```python
from build123d import *

# Parameters (mm, degrees)
F0_W     = 100
F0_H     = 100
F1_DEPTH = 100
F2_W     = 100
F2_H     = 20
F3_DEPTH = 40
F4_W     = 60.561549
F4_H     = 32.747179
F5_DEPTH = 100.001


with BuildPart() as f1:
    # F0 (on Top) → F1 (new body)
    with BuildSketch(Plane.XY):
        Rectangle(F0_W, F0_H)
    extrude(amount=F1_DEPTH)

    # F2 (on face) → F3 (join)
    with BuildSketch(Plane.XY.offset(100)):
        with Locations((0, 40)):
            Rectangle(F2_W, F2_H)
    extrude(amount=F3_DEPTH)

    # F4 (on face) → F5 (cut, through all)
    with BuildSketch(Plane.XZ.offset(50)):
        with Locations((-2.157872, 16.373589)):
            Rectangle(F4_W, F4_H)
    extrude(amount=-F5_DEPTH, mode=Mode.SUBTRACT)


solid = f1.part
```
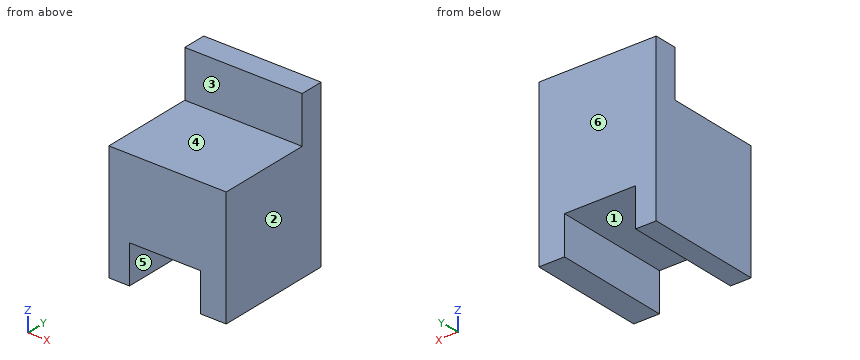
The model under review builds one solid part; all positions refer to its coordinate system, in mm. Face numbers are marked on the shaded views. A direction names the side the tool comes from. Coordinates: 2 decimals unless noted, no trailing zeros. Write each loop counter-clockwise with the first axis right and the second up, starting at its lowest first coordinate (ties: lowest second). Pieces come first, ordered by that corner, then holes.
1) To check wall thickness, follow probe 1 along X at (y, z) = (32, 21.5); probe 2 along Z at (x, y) = (-23, -11); probe 3 along Y at (x, z) = (-25, 128.5). State the ranges of each line that lie inside material, in increasing order.
2) We need section D-D on x = 14.5. State the section outline as (y, z) points.
3) We need section A-A on z = 21. State the section outline as (x, y) points, then the cut area to 3 significant figures.
4) We need section B-B on x = 32. State the section outline as (y, z) points.
5) Machinability: for the marked faces 4, 5 and 6, which of the approach directions +Z, -Z, +X, -X, +Y, -Y give a long, thin tool a straight path to every point of the face, cutting with its end or side? Answer none if there is none.
6) We need section C-C on y = -11. State the section outline as (x, z) points, then the cut area to 3 significant figures.
7) Clearance check with flat-ended pins moving along their axes: pin 1 Ø3 at (x, y) = (-30.5, -7) entering from +Z; pin 2 Ø12 at (x, y) = (20, 22.5) entering from -Z; pin 3 Ø5 at (x, z) = (14, 100.5) entering from -Y. State where each tip first meets the part, or that it passes through.
8) The part is to be moulded in two halves that separate along X. For the marked faces 1, 2 and 3, say which applies: pulls with the +X half, pulls with the -X half, needs draft (parallel to the pull), parting line crosses it, or undercut.
Answer list:
1. probe 1: x = -50 to -32.44, 28.12 to 50
1. probe 2: z = 32.75 to 100
1. probe 3: y = 30 to 50
2. outline: (-50, 32.75) - (50, 32.75) - (50, 140) - (30, 140) - (30, 100) - (-50, 100) - close
3. outline: (-50, -50) - (-32.44, -50) - (-32.44, 50) - (-50, 50) - close; (28.12, -50) - (50, -50) - (50, 50) - (28.12, 50) - close
3. area: 3,940 mm2
4. outline: (-50, 0) - (50, 0) - (50, 140) - (30, 140) - (30, 100) - (-50, 100) - close
5. face 4: +Z, +X, -X, -Y
5. face 5: -Z, +Y, -Y
5. face 6: +Z, -Z, +X, -X, +Y
6. outline: (-50, 0) - (-32.44, 0) - (-32.44, 32.75) - (28.12, 32.75) - (28.12, 0) - (50, 0) - (50, 100) - (-50, 100) - close
6. area: 8,020 mm2
7. pin 1: stops at z = 100
7. pin 2: stops at z = 32.75
7. pin 3: stops at y = -50
8. face 1: undercut
8. face 2: pulls with the +X half
8. face 3: needs draft
